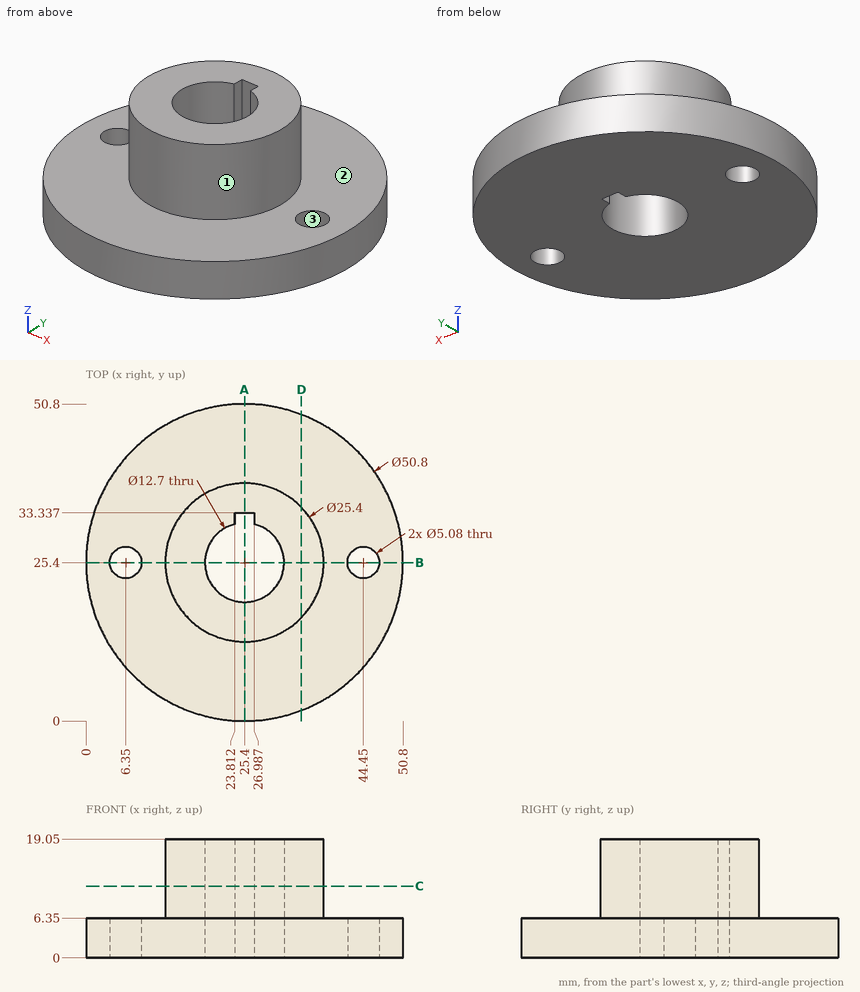
Input: dimensioned drawing with shaded views. Units: mm. Origin: part minimum x, y, z. Round coordinates to 2 decimals unless told otherwise and drop trailing zeros. Loops run counter-clockwise (first coordinate to the right, second up) from the corner with the lowest first, then second, coordinate; pieces in that order, holes last. Notation, with made-up numbers: M -40,-24.75 L -28,-24.75 A23 ccw -28,3.25 Z; hole C 55.25,-20 d1. An arc over 180 degrees is marked long. Return JSON: item names as keys, results as strings. Group by question number.
1. Material intervals for line 1 along Y through (x, z) = (25.4, 9.5); line 2 along Z through (x, y) = (46, 20); line 3 along Y through (x, z) = (21, 5.75) (1 decimal), sorted ascending. Write a range as from..to.
2. Section query A-A on x = 25.4. Output: boundary loops of the cut face in (y, z), and give its area (3 significant figures).
3. Section query B-B on y = 25.4. Output: boundary loops of the cut face in (x, z).
4. Pin query (flat end, axial travel): pin 1 (2 mm diameter, centred on y = 35, z = 3, fed in from -X); pin 2 (2 mm diameter, centred on y = 16.5, z = 11.5, fed in from +X) (1 decimal); pin 3 (8 mm diameter, centred on x = 6.35, y = 25.4, fed in from +Z); pin 4 (7.5 mm diameter, centred on x = 25.4, y = 25.4, fed in from -Z). Return the tip coordinate at first contact, or that it passes through.
5. Section query D-D on x = 34.5. Output: boundary loops of the cut face in (y, z), and give its area (3 significant figures).
6. Mould query, pull axis X, two halves, no side actions, for the marked faces 1, 2 and 3. Classes: released by +X, released by -X, zero draft, split by the parting line, or undercut.
7. Section query C-C on z = 11.5. Output: boundary loops of the cut face in (x, y), and give its area (3 significant figures).
Checks:
{
 "1": {"line 1": "y = 12.7..19.05, 33.34..38.1", "line 2": "z = 0..6.35", "line 3": "y = 0.4..20.8, 30..50.4"},
 "2": {"outline": "M 0,0 L 19.05,0 L 19.05,19.05 L 12.7,19.05 L 12.7,6.35 L 0,6.35 Z; M 33.34,0 L 50.8,0 L 50.8,6.35 L 38.1,6.35 L 38.1,19.05 L 33.34,19.05 Z", "area": "373 mm²"},
 "3": {"outline": "M 0,0 L 3.81,0 L 3.81,6.35 L 0,6.35 Z; M 8.89,0 L 19.05,0 L 19.05,19.05 L 12.7,19.05 L 12.7,6.35 L 8.89,6.35 Z; M 31.75,0 L 41.91,0 L 41.91,6.35 L 38.1,6.35 L 38.1,19.05 L 31.75,19.05 Z; M 46.99,0 L 50.8,0 L 50.8,6.35 L 46.99,6.35 Z"},
 "4": {"pin 1": "stops at x = 1.5", "pin 2": "stops at x = 35.3", "pin 3": "stops at z = 6.35", "pin 4": "passes through"},
 "5": {"outline": "M 1.69,0 L 49.11,0 L 49.11,6.35 L 34.26,6.35 L 34.26,19.05 L 16.54,19.05 L 16.54,6.35 L 1.69,6.35 Z", "area": "526 mm²"},
 "6": {"face 1": "split by the parting line", "face 2": "zero draft", "face 3": "undercut"},
 "7": {"outline": "C 25.4,25.4 d25.4; hole M 23.81,31.55 A6.35 ccw long 26.99,31.55 L 26.99,33.34 L 23.81,33.34 Z", "area": "375 mm²"}
}
